Geometry: final body of the model. Coordinates: model frame, mm. Face numbers are marked on the shaded views. A direction names the side the tool comes from. Give positions to 0.01 mm unless a question says otherwise; leave off trailing zeros. Loops run counter-clockwise (first coordinate to the right, second up) from the corner with the lowest first, then second, coordinate; pieces in that order, holes last.
```python
from build123d import *

# Parameters (mm, degrees)
F0_R     = 2.15265
F0_R_2   = 12.7
F1_DEPTH = 10.795
F2_R     = 14.2875
F3_DEPTH = 7.9375


with BuildPart() as f1:
    # F0 (on Top) → F1 (new body)
    with BuildSketch(Plane.XY):
        with BuildLine():
            Line((-17.005526, 3.96875), (-18.25625, 3.96875))
            ThreePointArc((-18.25625, 3.96875), (-22.225, 0), (-18.25625, -3.96875))
            Line((-18.25625, -3.96875), (-17.005526, -3.96875))
            ThreePointArc((-17.005526, -3.96875), (-12.347852, -12.347852), (-3.96875, -17.005526))
            Line((-3.96875, -17.005526), (-3.96875, -18.25625))
            ThreePointArc((-3.96875, -18.25625), (0, -22.225), (3.96875, -18.25625))
            Line((3.96875, -18.25625), (3.96875, -17.005526))
            ThreePointArc((3.96875, -17.005526), (12.347852, -12.347852), (17.005526, -3.96875))
            Line((17.005526, -3.96875), (18.25625, -3.96875))
            ThreePointArc((18.25625, -3.96875), (22.225, 0), (18.25625, 3.96875))
            Line((18.25625, 3.96875), (17.005526, 3.96875))
            ThreePointArc((17.005526, 3.96875), (12.347852, 12.347852), (3.96875, 17.005526))
            Line((3.96875, 17.005526), (3.96875, 18.25625))
            ThreePointArc((3.96875, 18.25625), (0, 22.225), (-3.96875, 18.25625))
            Line((-3.96875, 18.25625), (-3.96875, 17.005526))
            ThreePointArc((-3.96875, 17.005526), (-12.347852, 12.347852), (-17.005526, 3.96875))
        make_face()
        with Locations((0, -18.25625)):
            Circle(F0_R, mode=Mode.SUBTRACT)
        with Locations((-18.25625, 0)):
            Circle(F0_R, mode=Mode.SUBTRACT)
        Circle(F0_R_2, mode=Mode.SUBTRACT)
        with Locations((18.25625, 0)):
            Circle(F0_R, mode=Mode.SUBTRACT)
        with Locations((0, 18.25625)):
            Circle(F0_R, mode=Mode.SUBTRACT)
    extrude(amount=F1_DEPTH)

    # F2 (on face) → F3 (cut)
    with BuildSketch(Plane(origin=(0, 0, 0), x_dir=(1, 0, 0), z_dir=(0, 0, -1))):
        Circle(F2_R)
    extrude(amount=-F3_DEPTH, mode=Mode.SUBTRACT)


solid = f1.part
```
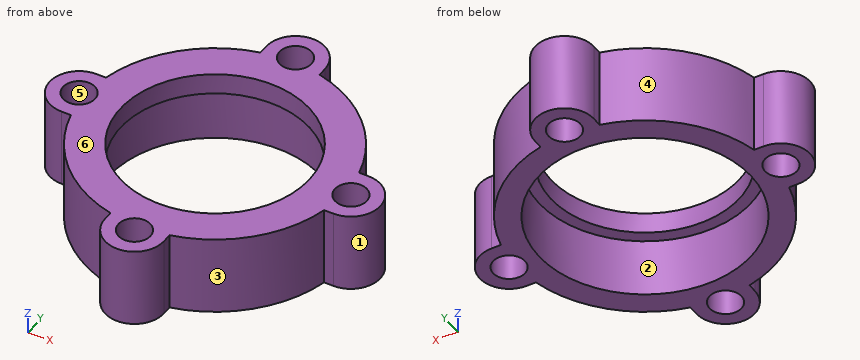
Q1. Section query D-D, the plane y = 11.5. Return loops of the section in (x, z) (1 decimal).
Q2. Pin query (flat end, axial travel): pin 1 Ø2 at (y, z) = (14.5, 3) entering from -X; pin 2 Ø23 at (x, y) = (0, 0) entering from +Z; pin 3 Ø0.6 at (y, z) = (17.5, 5) entering from -X; pin 4 Ø3 at (x, z) = (12, 1) entering from +Y. Return the tip coordinate at first contact, or that it passes through.
Q3. Mould query, pull axis X, two halves, no side actions, for the marked faces 3, 4, 5 and 6. Classes: +X half, -X half, draft (parallel to the pull), parting line (faces both ways), or undercut.
Q4. Section query A-A, the plane y = 0. Return loops of the section in (x, z) (1 decimal).
Q5. Material intervals for probe 1 along Y at (x, z) = (0, 3) (1 decimal); probe 2 along X at (y, z) = (0.5, 1); probe 3 along Y at (x, z) = (-5, 3.5), sorted ascending.
Q6. Section query C-C, the plane z = 5.75. Return loops of the section in (x, y) (1 decimal), and give its area (3 significant figures).
Q7. Reachability of the marked faces 1 and 2 from +Z, -Z, +X, -X, +Y, -Y: full face, straight path, thin tool, end or side. Return the list, or none.
Resolved:
1. outline: (-13.1, 0) - (-8.5, 0) - (-8.5, 7.9) - (-5.4, 7.9) - (-5.4, 10.8) - (-13.1, 10.8) - close; (5.4, 7.9) - (8.5, 7.9) - (8.5, 0) - (13.1, 0) - (13.1, 10.8) - (5.4, 10.8) - close
2. pin 1: stops at x = -11.08
2. pin 2: passes through
2. pin 3: stops at x = -3.97
2. pin 4: stops at y = 13.95
3. face 3: +X half
3. face 4: -X half
3. face 5: undercut
3. face 6: draft
4. outline: (-22.2, 0) - (-20.4, 0) - (-20.4, 10.8) - (-22.2, 10.8) - close; (-16.1, 0) - (-14.3, 0) - (-14.3, 7.9) - (-12.7, 7.9) - (-12.7, 10.8) - (-16.1, 10.8) - close; (12.7, 7.9) - (14.3, 7.9) - (14.3, 0) - (16.1, 0) - (16.1, 10.8) - (12.7, 10.8) - close; (20.4, 0) - (22.2, 0) - (22.2, 10.8) - (20.4, 10.8) - close
5. probe 1: y = -22.2 to -20.4, -16.1 to -14.3, 14.3 to 16.1, 20.4 to 22.2
5. probe 2: x = -22.19 to -20.35, -16.16 to -14.28, 14.28 to 16.16, 20.35 to 22.19
5. probe 3: y = -16.73 to -13.38, 13.38 to 16.73
6. outline: (-18.3, -4) - (-17, -4) arc R17.5 ccw to (-4, -17) - (-4, -18.3) arc R4 ccw to (4, -18.3) - (4, -17) arc R17.5 ccw to (17, -4) - (18.3, -4) arc R4 ccw to (18.3, 4) - (17, 4) arc R17.5 ccw to (4, 17) - (4, 18.3) arc R4 ccw to (-4, 18.3) - (-4, 17) arc R17.5 ccw to (-17, 4) - (-18.3, 4) arc R4 ccw to start; hole circle Ø4.3 at (-18.3, 0); hole circle Ø28.6 at (0, 0); hole circle Ø4.3 at (0, -18.3); hole circle Ø4.3 at (0, 18.3); hole circle Ø4.3 at (18.3, 0)
6. area: 387 mm2
7. face 1: +Z, -Z, +X
7. face 2: -Z
